from build123d import *

# Parameters (mm, degrees)
ESQUISSE1_W        = 3.5
ESQUISSE1_H        = 5
ESQUISSE1_W_2      = 5
ESQUISSE1_H_2      = 3.5
ESQUISSE1_W_3      = 4
BOSS_EXTRU_1_DEPTH = 260


with BuildPart() as part:
    # Esquisse1 → Boss.-Extru.1 (new body)
    with BuildSketch(Plane.XY):
        Polygon((7.5, 16), (7.5, 20), (0, 20), (4, 16), align=None)
        Polygon((4, 16), (0, 20), (0, 12.5), (4, 12.5), align=None)
        Polygon((4, 7.5), (0, 7.5), (0, 0), (4, 4), align=None)
        Polygon((0, 0), (7.5, 0), (7.5, 4), (4, 4), align=None)
        Polygon((4, 4), (7.5, 7.5), (4, 7.5), align=None)
        Polygon((7.5, 4), (7.5, 7.5), (4, 4), align=None)
        Polygon((4, 12.5), (7.5, 12.5), (4, 16), align=None)
        Polygon((7.5, 12.5), (7.5, 16), (4, 16), align=None)
        with Locations((5.75, 10)):
            Rectangle(ESQUISSE1_W, ESQUISSE1_H)
        Polygon((7.5, 7.5), (10, 10), (7.5, 12.5), align=None)
        Polygon((10, 10), (12.5, 12.5), (7.5, 12.5), align=None)
        Polygon((12.5, 7.5), (12.5, 12.5), (10, 10), align=None)
        Polygon((12.5, 7.5), (10, 10), (7.5, 7.5), align=None)
        Polygon((16, 4), (12.5, 7.5), (12.5, 4), align=None)
        Polygon((16, 4), (16, 7.5), (12.5, 7.5), align=None)
        Polygon((20, 0), (20, 7.5), (16, 7.5), (16, 4), align=None)
        with Locations((10, 14.25)):
            Rectangle(ESQUISSE1_W_2, ESQUISSE1_H_2)
        with Locations((14.25, 10)):
            Rectangle(ESQUISSE1_W, ESQUISSE1_H)
        Polygon((12.5, 12.5), (16, 16), (12.5, 16), align=None)
        Polygon((16, 16), (20, 20), (12.5, 20), (12.5, 16), align=None)
        Polygon((16, 12.5), (16, 16), (12.5, 12.5), align=None)
        Polygon((20, 12.5), (20, 20), (16, 16), (16, 12.5), align=None)
        Polygon((12.5, 0), (20, 0), (16, 4), (12.5, 4), align=None)
        with Locations((10, 5.75)):
            Rectangle(ESQUISSE1_W_2, ESQUISSE1_H_2)
        with Locations((18, 10)):
            Rectangle(ESQUISSE1_W_3, ESQUISSE1_H)
        with Locations((22, 10)):
            Rectangle(ESQUISSE1_W_3, ESQUISSE1_H)
        Polygon((24, 16), (20, 20), (20, 12.5), (24, 12.5), align=None)
        Polygon((27.5, 20), (20, 20), (24, 16), (27.5, 16), align=None)
        Polygon((27.5, 12.5), (24, 16), (24, 12.5), align=None)
        Polygon((27.5, 16), (24, 16), (27.5, 12.5), align=None)
        with Locations((25.75, 10)):
            Rectangle(ESQUISSE1_W, ESQUISSE1_H)
        Polygon((27.5, 7.5), (24, 7.5), (24, 4), align=None)
        Polygon((24, 7.5), (20, 7.5), (20, 0), (24, 4), align=None)
        Polygon((24, 4), (20, 0), (27.5, 0), (27.5, 4), align=None)
        Polygon((27.5, 4), (27.5, 7.5), (24, 4), align=None)
        with Locations((30, 5.75)):
            Rectangle(ESQUISSE1_W_2, ESQUISSE1_H_2)
        Polygon((36, 4), (32.5, 7.5), (32.5, 4), align=None)
        Polygon((36, 7.5), (32.5, 7.5), (36, 4), align=None)
        Polygon((40, 0), (40, 7.5), (36, 7.5), (36, 4), align=None)
        Polygon((32.5, 4), (32.5, 0), (40, 0), (36, 4), align=None)
        with Locations((34.25, 10)):
            Rectangle(ESQUISSE1_W, ESQUISSE1_H)
        Polygon((32.5, 12.5), (30, 10), (32.5, 7.5), align=None)
        Polygon((32.5, 7.5), (30, 10), (27.5, 7.5), align=None)
        Polygon((30, 10), (27.5, 12.5), (27.5, 7.5), align=None)
        Polygon((32.5, 12.5), (27.5, 12.5), (30, 10), align=None)
        Polygon((36, 16), (32.5, 12.5), (36, 12.5), align=None)
        Polygon((36, 16), (32.5, 16), (32.5, 12.5), align=None)
        Polygon((40, 20), (32.5, 20), (32.5, 16), (36, 16), align=None)
        Polygon((40, 12.5), (40, 20), (36, 16), (36, 12.5), align=None)
        with Locations((30, 14.25)):
            Rectangle(ESQUISSE1_W_2, ESQUISSE1_H_2)
    extrude(amount=BOSS_EXTRU_1_DEPTH)


solid = part.part
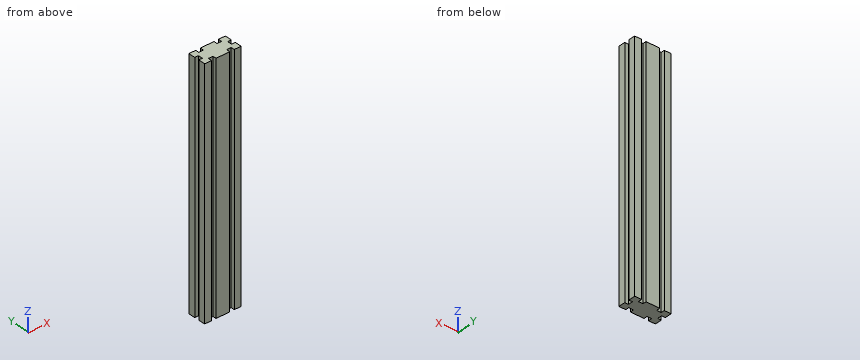
The listing builds one solid part. Answer for the finished solid, in the listing's coordinates (mm). Round coordinates to 2 decimals unless told otherwise and drop trailing zeros. Write each loop counter-clockwise with the first axis right and the second up, starting at its lowest first coordinate (ties: lowest second). Pieces come first, ordered by that corner, then holes. Notation, with made-up numbers: M 38,-29 L 46,-29 A17 cw 46,4 Z; hole C -0.75,19 d1. An arc over 180 degrees is marked long. Write each question's results on one line, items separated by ' | '. Start each with the question number.
(1) The part is cut by section A-A, the plane z = 206. Write down the section's boundary in (x, y).
(2) Find the intervals of material crossed by line 1 (X direction, y = 3.25, z = 164.5); line 2 (Y direction, x = 36.5, z = 198); line 3 (X direction, y = 9, z = 230.5), in increasing order.
(3) Each of these flat-tipped pins is pushed along its axis until it touches: P1, Ø2.5, axis at y = 11, z = 110.5, coming from the -X side; P2, Ø1.5, axis at y = 10.5, z = 93, coming from the +X side. Where does it stop, or does it pass through?
Worked answers:
1) outline: M 0,0 L 7.5,0 L 7.5,4 L 12.5,4 L 12.5,0 L 27.5,0 L 27.5,4 L 32.5,4 L 32.5,0 L 40,0 L 40,7.5 L 36,7.5 L 36,12.5 L 40,12.5 L 40,20 L 32.5,20 L 32.5,16 L 27.5,16 L 27.5,20 L 12.5,20 L 12.5,16 L 7.5,16 L 7.5,20 L 0,20 L 0,12.5 L 4,12.5 L 4,7.5 L 0,7.5 Z
2) line 1: x = 0 to 7.5, 12.5 to 27.5, 32.5 to 40 | line 2: y = 0 to 7.5, 12.5 to 20 | line 3: x = 4 to 36
3) P1: stops at x = 4 | P2: stops at x = 36
